Design review of the part built by this model. Coordinates are the model's own, in mm. A direction names the side the tool comes from. Coordinates: 2 decimals unless noted, no trailing zeros. Order: outer loops, then holes, each group sorted by start corner. A loop starts at its lowest first (then second) coordinate and runs counter-clockwise, first axis right, second up. Notation, with made-up numbers: (29.25, 8) -> (76.25, 8) arc R18 cw to (76.25, 43) -> close; hole circle Ø6 at (49.5, 7). An arc over 180 degrees is marked (long way). Write item = value, one per line.
Autodesk Inventor part; units mm, degrees
ref_plane "Work Plane1" through (104.775, 0, 0) normal (0, 0, -1) x (1, 0, 0)
ref_plane "YZ Plane" through (0, 0, 0) normal (1, 0, 0) x (0, 1, 0)
ref_plane "XZ Plane" through (0, 0, 0) normal (0, 1, 0) x (-1, 0, 0)
sketch "Skizze1" plane through (0, 0, 0) normal (0, 0, 1) x (1, 0, 0)
  line L0 (8, 0) -> (8, 2.5)
  line L1 (8, 2.5) -> (5.5, 2.5)
  line L2 (5.5, 2.5) -> (5.0092, 2.5)
  line L3 (0, 4.715) -> (0, 1.7321)
  line L4 (0, 1.7321) -> (1.9, 1.7321)
  line L5 (1.9, 1.7321) -> (2.9, 0)
  line L6 (2.9, 0) -> (8, 0)
  line L7 (0, 4.715) -> (0.885, 4.715)
  line L8 (0.885, 4.715) -> (3.1, 2.5)
  line L9 (5.0092, 2.5) -> (3.1, 2.5)
  line L10 (5.5, 2.5) -> (3.1, 2.5) construction
  line L11 (3.1, 2.5) -> (3.1, 2.5)
  line L12 (-1.6, 0) -> (9.6, 0)
  line L13 (0, -0.943) -> (0, 5.658)
  dimension "d0" = 8
  dimension "d1" = 2.5
  dimension "d2" = 1.9
  dimension "d3" = 5
  dimension "d6" = 3.1
  dimension "d7" = 45
  dimension "d8" = 3.4641
  dimension "d9" = 60
  dimension "d10" = 9.43
  dimension "d11" = 5
  dimension "d12" = 0.4908
revolve "Körper" add sketch "Skizze1" angle 360 about axis through (2.9, 0, 0) along (1, 0, 0) contours L6 L5 L4 L3 L7 L8 L9 L2 L1 L0
sketch "Skizze2" plane through (0, 0, 0) normal (-1, 0, 0) x (0, 0, 1)
  circle A0 centre (0, 0) radius 1.7321
  line L0 (0, -6.601) -> (0, 6.601)
  line L1 (-6.601, 0) -> (6.601, 0)
  line L2 (1.7321, 0) -> (0.866, -1.5)
  line L3 (0.866, -1.5) -> (-0.866, -1.5)
  line L4 (-0.866, -1.5) -> (-1.7321, 0)
  line L5 (-1.7321, 0) -> (-0.866, 1.5)
  line L6 (-0.866, 1.5) -> (0.866, 1.5)
  line L7 (0.866, 1.5) -> (1.7321, 0)
  point P0 (0, 1.7321)
extrude "Loch" add sketch "Skizze2" against normal up to next contours L7 A0 | A0 L2 | L6 L0 A0 | A0 L0 L3 | L0 L6 A0 | A0 L3 L0 | L4 A0 | A0 L5
thread "Gewinde"
chamfer "Fase1" distance 0.4908 distance2 0.4908 1 edges at (8, -2.5, 0) measured on face at (8, 0.4809, 1.5312)
ref_plane "Work Plane1" through (104.775, 0, 0) normal (0, 0, -1) x (1, 0, 0)
equation "\"d15\" = GEL"
equation "\"d17\" = -0.5 * SPD + 0.5 * GD"
equation "\"d18\" = GUL"
equation "\"d0\" = NLG"
equation "\"d1\" = GEL"
equation "\"d2\" = INTI"
equation "\"d3\" = GD"
equation "\"d6\" = KOH"
equation "\"d7\" = 0.5 * SEWI"
equation "\"d8\" = 1.1547 * SW"
equation "\"d10\" = KOD"
equation "\"d11\" = BDM"
equation "\"d12\" = GAL"
equation "\"NLG\" = 8"
equation "\"INTI\" = 1.9"
equation "\"GEL\" = 2.5"
equation "\"GAL\" = 0.61345 * PTC"
equation "\"KOH\" = 3.1"
equation "\"KOD\" = 9.43"
equation "\"GUL\" = 0.61345 * PTC"
equation "\"SPD\" = NND - 1.2269 * PTC"
equation "\"BDM\" = NND"
equation "\"GD\" = NND"
equation "\"SEWI\" = 90deg"
equation "\"SW\" = 3"
equation "\"TOA\" = 30deg"
equation "\"GD1\" = THREADDIA - 1.2269 * PTC"
equation "\"EPV\" = 5.5"
equation "\"THREADDIA\" = 5"
equation "\"PTC\" = 0.8"
equation "\"NND\" = 5"
equation "\"E0\" = 3.47"
properties part number "ISO 10642  - M5  x  8" material "Stahl"
(1) The part is to be moulded in two halves that separate along Z. For faces 4 (the cylindrical face through (0.449, -0.614, 4.675)), 5 (the flat face through (8, 0, 0)), 6 (the flat face through (1.003, 0.761, 1.293)), say which applies: released by +Z, released by -Z, zero draft, split by the parting line, or undercut.
Report:
face_4 = split by the parting line
face_5 = zero draft
face_6 = undercut
(2) For faces 1 (the flat face through (0, 0, 2)), 2 (the flat face through (1, 1.5, 0)), 3 (the cylindrical face through (5.27, -0.54, 2.44)), list the 3-axis set-ups (+Z, -Z, +X, -X, +Y, -Y) from which the entire face can be reached by the end or side of a thin tool; tool diameter is ignored.
Report:
face_1 = +Z, -Z, -X, +Y, -Y
face_2 = -X
face_3 = +X
(3) We need section A-A (x = 3.25). Write out the cut boundary in (y, z), and give its area (3 significant figures).
Report:
outline = circle Ø5 at (0, 0)
area = 19.6 mm²
(4) For L1, parallel to Z at x = 7.25, y = 0; L2, parallel to Y at x = 3, z = -1.75; L3, parallel to Y at x = 0.5, z = 2.5, list the stretches that pass through material, from the lowest coordinate up.
Report:
L1 = -2.5 to 2.5
L2 = -1.92 to 1.92
L3 = -4 to 4
(5) Insertion check: pin 1 (1.5 mm diameter, centred on x = 7, z = -2, fed in from -Y); pin 2 (0.5 mm diameter, centred on x = 0.5, z = 0.5, fed in from +Y); pin 3 (3 mm diameter, centred on x = 4, y = -3, fed in from +Z). Each pin has a flat end and moves straight along its axis. Give the tip position at first contact, or say it passes through.
Report:
pin_1 = -2.17
pin_2 = 4.71
pin_3 = 2
